from build123d import *

# Parameters (mm, degrees)
SKETCH1_R        = 3.175
EXTRUSION1_DEPTH = 25.4


with BuildPart() as part:
    # Sketch1 → Extrusion1 (new body)
    with BuildSketch(Plane.XY):
        Polygon((6.35, 0), (63.5, 0), (63.5, 21.59), (59.69, 21.59), (6.35, 21.59), align=None)
        with Locations((12.693410129, 12.073465073)):
            Circle(SKETCH1_R, mode=Mode.SUBTRACT)
        Polygon((14.928610129, 28.154355163), (12.693410129, 21.59), (16.503410129, 21.59), (19.373610129, 21.59), (17.138410129, 28.154355163), (16.033510129, 28.154355163), align=None)
        Polygon((25.241010129, 28.154355163), (23.005810129, 21.59), (29.686010129, 21.59), (27.450810129, 28.154355163), (26.345910129, 28.154355163), align=None)
        Polygon((59.69, 21.59), (60.623210129, 21.59), (58.388010129, 28.154355163), (57.283110129, 28.154355163), (56.178210129, 28.154355163), (53.943010129, 21.59), align=None)
        Polygon((43.630610129, 21.59), (50.310810129, 21.59), (48.075610129, 28.154355163), (46.970710129, 28.154355163), (45.865810129, 28.154355163), align=None)
        Polygon((39.996666979, 21.59), (39.998410129, 21.59), (37.763210129, 28.154355163), (36.658310129, 28.154355163), (35.553410129, 28.154355163), (33.318210129, 21.59), (36.186666979, 21.59), align=None)
    extrude(amount=EXTRUSION1_DEPTH)


solid = part.part
CAD build for the part. Positions are in the model's coordinates, mm. A direction names the side the tool comes from. Give positions to 0.01 mm unless a question says otherwise; leave off trailing zeros. Write each loop counter-clockwise with the first axis right and the second up, starting at its lowest first coordinate (ties: lowest second). Pieces come first, ordered by that corner, then holes. Notation, with made-up numbers: M -25,17 L 3,17 A20 ccw 3,36 Z; hole C 23,73.5 d6. An arc over 180 degrees is marked long. Put each result on its own line as item: value. Start each with the question number.
(1) Probe L1, parallel to X at y = 24.5, z = 15.25; L2, parallel to X at y = 25, z = 5.5; L3, parallel to Y at x = 50.5, z = 23. List the from-to ranges inside material, lowest first.
(2) Band-saw the part on D-D, the plane x = 55.5. Write the cut outline in (y, z).
(3) Band-saw the part on C-C, the plane z = 7.75. Write the cut outline in (x, y) (3 decimals).
(4) Which spindle directions (+Z, -Z, +X, -X, +Y, -Y) get a long thin tool onto all of the face, cutting with end or side? Do faces 1 (the face through (35, 11, 25.4)), 2 (the face through (62, 21.59, 13)), 3 (the face through (55.076, 24.918, 12.522)). Say none if no direction does.
(5) Band-saw the part on A-A, the plane x = 14. Write the cut outline in (y, z).
(6) Flat gauge pin, fed straight in: pin 1 Ø5 at (x, z) = (9.5, 12.5) entering from +Y. Where does the tip first touch, or does it go through?
(7) Band-saw the part on B-B, the plane y = 11.5. Write the cut outline in (x, z).
(8) Mould opens along Y. For faces 4 (the face through (35, 0, 13)), 5 (the face through (59.52, 24.83, 12.52)), 6 (the face through (15.72, 13.03, 12.52)) say: +Y half, -Y half, draft (parallel to the pull), parting line (faces both ways), or undercut.
Response values:
1. L1: x = 13.68 to 18.38, 24 to 28.7, 34.31 to 39.01, 44.62 to 49.32, 54.93 to 59.63
1. L2: x = 13.85 to 18.21, 24.17 to 28.52, 34.48 to 38.84, 44.79 to 49.15, 55.1 to 59.46
1. L3: y = 0 to 21.59
2. outline: M 0,0 L 26.16,0 L 26.16,25.4 L 0,25.4 Z
3. outline: M 6.35,0 L 63.5,0 L 63.5,21.59 L 60.623,21.59 L 58.388,28.154 L 56.178,28.154 L 53.943,21.59 L 50.311,21.59 L 48.076,28.154 L 45.866,28.154 L 43.631,21.59 L 39.998,21.59 L 37.763,28.154 L 35.553,28.154 L 33.318,21.59 L 29.686,21.59 L 27.451,28.154 L 25.241,28.154 L 23.006,21.59 L 19.374,21.59 L 17.138,28.154 L 14.929,28.154 L 12.693,21.59 L 6.35,21.59 Z; hole C 12.693,12.073 d6.35
4. face 1: +Z, +X, -X, +Y, -Y
4. face 2: +Z, -Z, +X, +Y
4. face 3: +Z, -Z, +Y
5. outline: M 0,0 L 9.18,0 L 9.18,25.4 L 0,25.4 Z; M 14.97,0 L 25.43,0 L 25.43,25.4 L 14.97,25.4 Z
6. pin 1: stops at y = 21.59
7. outline: M 6.35,0 L 9.57,0 L 9.57,25.4 L 6.35,25.4 Z; M 15.82,0 L 63.5,0 L 63.5,25.4 L 15.82,25.4 Z
8. face 4: -Y half
8. face 5: +Y half
8. face 6: undercut
